from build123d import *

# Parameters (mm, degrees)
SKETCH1_W           = 230
SKETCH1_H           = 90
BOSS_EXTRUDE1_DEPTH = 5
CUT_EXTRUDE1_REACH  = 125.592
SKETCH2_R           = 11
SKETCH2_R_2         = 16.75
CUT_EXTRUDE2_REACH  = 125.592
SKETCH3_R           = 4.65
SKETCH3_R_2         = 4.8
MOVE_FACE1_BY       = 2
SKETCH5_W           = 20.50990482
SKETCH5_H           = 126.384873773
CUT_EXTRUDE3_DEPTH  = 5
SKETCH6_W           = 30
SKETCH6_H           = 5
BOSS_EXTRUDE3_DEPTH = 5
CUT_EXTRUDE4_DEPTH  = 10
BOSS_EXTRUDE4_DEPTH = 5
SKETCH8_R           = 20
SKETCH8_R_2         = 4.65
SKETCH8_R_3         = 4.8
SKETCH8_R_4         = 11
CUT_EXTRUDE5_DEPTH  = 5


with BuildPart() as part:
    # Sketch1 → Boss-Extrude1 (new body)
    with BuildSketch(Plane.XY):
        Rectangle(SKETCH1_W, SKETCH1_H)
    extrude(amount=BOSS_EXTRUDE1_DEPTH)

    # Sketch2 → Cut-Extrude1 (cut, up to next)
    with BuildSketch(Plane.XY.offset(5), mode=Mode.PRIVATE) as cut_extrude1_sk1:
        with Locations((-20.95, 10)):
            Circle(SKETCH2_R)
    cut_extrude1_tool1 = extrude(cut_extrude1_sk1.sketch, amount=-CUT_EXTRUDE1_REACH, mode=Mode.PRIVATE) & part.part
    # Sketch2 → Cut-Extrude1 (cut, up to next)
    with BuildSketch(Plane.XY.offset(5), mode=Mode.PRIVATE) as cut_extrude1_sk2:
        with Locations((20.95, 10)):
            Circle(SKETCH2_R)
    cut_extrude1_tool2 = extrude(cut_extrude1_sk2.sketch, amount=-CUT_EXTRUDE1_REACH, mode=Mode.PRIVATE) & part.part
    # Sketch2 → Cut-Extrude1 (cut, up to next)
    with BuildSketch(Plane.XY.offset(5), mode=Mode.PRIVATE) as cut_extrude1_sk3:
        with Locations((49.976927154, -10)):
            Circle(SKETCH2_R_2)
    cut_extrude1_tool3 = extrude(cut_extrude1_sk3.sketch, amount=-CUT_EXTRUDE1_REACH, mode=Mode.PRIVATE) & part.part
    add(cut_extrude1_tool1.solids().sort_by_distance((-20.95, 10, 5))[0], mode=Mode.SUBTRACT)
    add(cut_extrude1_tool2.solids().sort_by_distance((20.95, 10, 5))[0], mode=Mode.SUBTRACT)
    add(cut_extrude1_tool3.solids().sort_by_distance((49.976927, -10, 5))[0], mode=Mode.SUBTRACT)

    # Sketch3 → Cut-Extrude2 (cut, up to next)
    with BuildSketch(Plane(origin=(0, 0, 0), x_dir=(-1, 0, 0), z_dir=(0, 0, -1)), mode=Mode.PRIVATE) as cut_extrude2_sk1:
        with Locations((-42.861480484, 27.315297382)):
            Circle(SKETCH3_R)
    cut_extrude2_tool1 = extrude(cut_extrude2_sk1.sketch, amount=-CUT_EXTRUDE2_REACH, mode=Mode.PRIVATE) & part.part
    # Sketch3 → Cut-Extrude2 (cut, up to next)
    with BuildSketch(Plane(origin=(0, 0, 0), x_dir=(-1, 0, 0), z_dir=(0, 0, -1)), mode=Mode.PRIVATE) as cut_extrude2_sk2:
        with Locations((-88.015918911, -8.560303387)):
            Circle(SKETCH3_R)
    cut_extrude2_tool2 = extrude(cut_extrude2_sk2.sketch, amount=-CUT_EXTRUDE2_REACH, mode=Mode.PRIVATE) & part.part
    # Sketch3 → Cut-Extrude2 (cut, up to next)
    with BuildSketch(Plane(origin=(0, 0, 0), x_dir=(-1, 0, 0), z_dir=(0, 0, -1)), mode=Mode.PRIVATE) as cut_extrude2_sk3:
        with Locations((-16.935196723, -27.604446885)):
            Circle(SKETCH3_R_2)
    cut_extrude2_tool3 = extrude(cut_extrude2_sk3.sketch, amount=-CUT_EXTRUDE2_REACH, mode=Mode.PRIVATE) & part.part
    add(cut_extrude2_tool1.solids().sort_by_distance((42.86148, 27.315297, 0))[0], mode=Mode.SUBTRACT)
    add(cut_extrude2_tool2.solids().sort_by_distance((88.015919, -8.560303, 0))[0], mode=Mode.SUBTRACT)
    add(cut_extrude2_tool3.solids().sort_by_distance((16.935197, -27.604447, 0))[0], mode=Mode.SUBTRACT)

    # Move Face1: a face moved outward by 2.0
    extrude(part.faces().sort_by_distance((0, 45, 2.5))[0], amount=MOVE_FACE1_BY, dir=(0, 1, 0))

    # Sketch5 → Cut-Extrude3 (cut)
    with BuildSketch(Plane(origin=(0, 0, 0), x_dir=(-1, 0, 0), z_dir=(0, 0, -1))):
        with Locations((104.74504759, -16.192436887)):
            Rectangle(SKETCH5_W, SKETCH5_H)
    extrude(amount=-CUT_EXTRUDE3_DEPTH, mode=Mode.SUBTRACT)

    # Sketch6 → Boss-Extrude3 (add)
    with BuildSketch(Plane(origin=(0, 0, 0), x_dir=(-1, 0, 0), z_dir=(0, 0, -1))):
        with Locations((5.391218518, -47.5)):
            Rectangle(SKETCH6_W, SKETCH6_H)
        with Locations((75.782437035, -47.5)):
            Rectangle(SKETCH6_W, SKETCH6_H)
        with Locations((-65, -47.5)):
            Rectangle(SKETCH6_W, SKETCH6_H)
    extrude(amount=-BOSS_EXTRUDE3_DEPTH)

    # Sketch7 → Cut-Extrude4 (cut)
    with BuildSketch(Plane.XY.offset(5)):
        Polygon((-42.686827777, -45), (-42.686827777, -37), (-44.136827777, -37), (-44.136827777, -33.5), (-42.686827777, -33.5), (-42.686827777, -27), (-38.486827777, -27), (-38.486827777, -33.5), (-37.036827777, -33.5), (-37.036827777, -37), (-38.486827777, -37), (-38.486827777, -45), align=None)
        Polygon((97.5, -45), (97.5, -37), (96.05, -37), (96.05, -33.5), (97.5, -33.5), (97.5, -27), (101.7, -27), (101.7, -33.5), (103.15, -33.5), (103.15, -37), (101.7, -37), (101.7, -45), align=None)
        Polygon((115, 24.402956743), (107, 24.402956743), (107, 22.952956743), (103.5, 22.952956743), (103.5, 24.402956743), (97, 24.402956743), (97, 28.602956743), (103.5, 28.602956743), (103.5, 30.052956743), (107, 30.052956743), (107, 28.602956743), (115, 28.602956743), align=None)
        Polygon((-62.609520372, 47), (-62.609520372, 39), (-61.159520372, 39), (-61.159520372, 35.5), (-62.609520372, 35.5), (-62.609520372, 29), (-66.809520372, 29), (-66.809520372, 35.5), (-68.259520372, 35.5), (-68.259520372, 39), (-66.809520372, 39), (-66.809520372, 47), align=None)
    extrude(amount=-CUT_EXTRUDE4_DEPTH, mode=Mode.SUBTRACT)

    # Sketch9 → Boss-Extrude4 (add)
    with BuildSketch(Plane.XY.offset(5)):
        Polygon((-39.58489376, 23.410750341), (-37.52309363, -9.578051742), (-6.596091677, -20.917952458), (6.599429156, -35.969093408), (51.752852007, -37.618533512), (87.628174272, -20.917952458), (101.85459517, 0), (47.084922834, 37.249172102), align=None)
    extrude(amount=-BOSS_EXTRUDE4_DEPTH)

    # Sketch8 → Cut-Extrude5 (cut)
    with BuildSketch(Plane.XY.offset(5)):
        with Locations((54.21355411, -11.517627108)):
            Circle(SKETCH8_R)
        with Locations((42.861480484, 27.315297382)):
            Circle(SKETCH8_R_2)
        with Locations((88.015918911, -8.560303387)):
            Circle(SKETCH8_R_2)
        with Locations((16.935196723, -27.604446885)):
            Circle(SKETCH8_R_3)
        with Locations((20.95, 10)):
            Circle(SKETCH8_R_4)
        with Locations((-20.95, 10)):
            Circle(SKETCH8_R_4)
    extrude(amount=-CUT_EXTRUDE5_DEPTH, mode=Mode.SUBTRACT)


solid = part.part
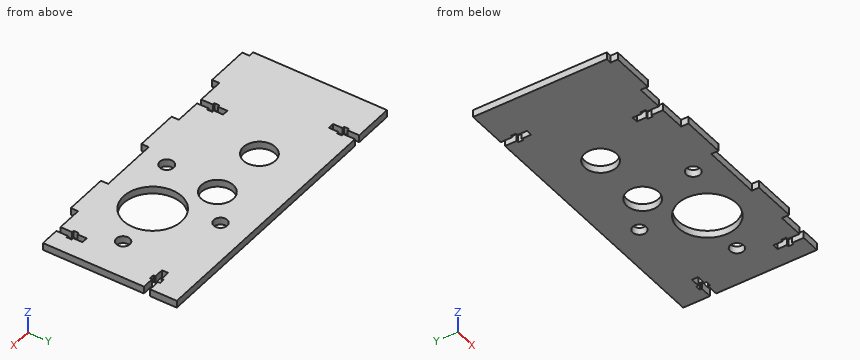
CAD build for the part. Positions are in the model's coordinates, mm. Give positions to 0.01 mm unless a question says otherwise; leave off trailing zeros. Loops run counter-clockwise (first coordinate to the right, second up) from the corner with the lowest first, then second, coordinate; pieces in that order, holes last. Notation, with made-up numbers: M 79,-21.5 L 123,-21.5 A19 cw 123,5.5 Z; hole C 46.5,-30.5 d3. An arc over 180 degrees is marked long. Answer in a Markdown table with one row per item. Add a question column.
Item 1: Probe probe 1 along X at (y, z) = (-41, 2.55); probe 2 along X at (y, z) = (17.5, 3.95); probe 3 along X at (y, z) = (36, 3.9). List the from-to ranges inside material, lowest first.
Item 2: Band-saw the part on A-A on y = -6. Give the cut face in (x, z).
Item 3: Drop flat-ended pins along their axis: P1, Ø1.5, axis at y = -48, z = 1.5, coming from the +X side; P2, Ø1.5, axis at x = -54.5, z = 3.5, coming from the -Y side; P3, Ø4, axis at x = -35.5, y = 16.5, coming from the -Z side. Give the stop position or say it passes through.
Item 4: Band-saw the part on B-B on z = 2.95. Give the number of separate pieces and of enclosed holes in the cut face, then the cut area to 3 significant figures.
Reply:
| question | item | result |
|---|---|---|
| 1 | probe 1 | x = -94.49 to -42.69, -38.49 to 97.5, 101.7 to 115 |
| 1 | probe 2 | x = -94.49 to -29, -12.9 to 12.9, 29 to 115 |
| 1 | probe 3 | x = -94.49 to -68.26, -61.16 to 115 |
| 2 | outline | M -94.49,0 L 34.99,0 L 34.99,5 L -94.49,5 Z; M 73.44,0 L 84.13,0 L 84.13,5 L 73.44,5 Z; M 91.9,0 L 115,0 L 115,5 L 91.9,5 Z |
| 3 | P1 | stops at x = 80 |
| 3 | P2 | stops at y = -45 |
| 3 | P3 | stops at z = 0 |
| 4 | separate pieces | 1 |
| 4 | enclosed holes | 6 |
| 4 | area | 17,200 mm^2 |
